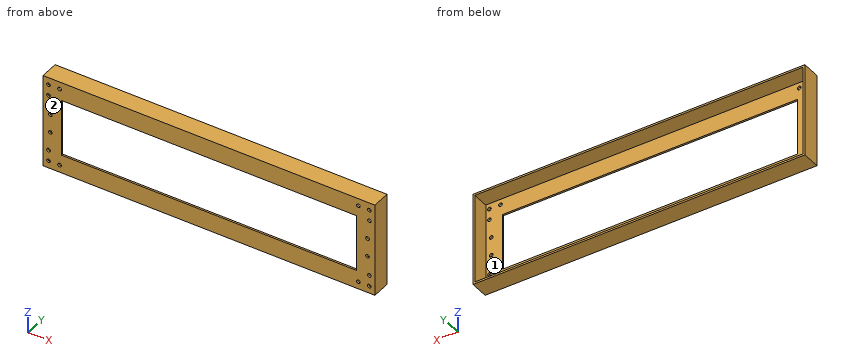
from build123d import *

# Parameters (mm, degrees)
CUT_EXTRUDE1_DEPTH      = 472.899618563
CUT_EXTRUDE1_DEPTH_BACK = 472.899618563
SKETCH5_R               = 5


with BuildPart() as part:
    # Sweep3: sweep along a path in Sketch1
    with BuildLine(Plane(origin=(0, 0, 0), x_dir=(1, 0, 0), z_dir=(0, 1, 0))) as sweep3_path:
        Line((-450, -125), (450, -125))
        Line((450, -125), (450, 125))
        Line((450, 125), (-450, 125))
        Line((-450, 125), (-450, -125))
    # Sketch2 → Sweep3 (sweep)
    with BuildSketch(Plane.XY):
        Polygon((402, -2.5), (452, -2.5), (452, 47.5), (447, 47.5), (447, 2.5), (402, 2.5), align=None)
    sweep(path=sweep3_path.line, transition=Transition.RIGHT)

    # Sketch5 → Cut-Extrude1 (cut, two sides: drawn at the far end of the back side and taken through both)
    with BuildSketch(Plane(origin=(0, 0, 0), x_dir=(1, 0, 0), z_dir=(0, 1, 0)).offset(-CUT_EXTRUDE1_DEPTH_BACK)):
        with Locations((-437, 107)):
            Circle(SKETCH5_R)
        with Locations(Location((-407, 107, 0), (0, 0, 270))):
            Circle(SKETCH5_R)
        with Locations(Location((-432, 25, 0), (0, 0, 270))):
            Circle(SKETCH5_R)
        with Locations(Location((-437, 77, 0), (0, 0, 270))):
            Circle(SKETCH5_R)
        with Locations(Location((-407, -107, 0), (0, 0, 270))):
            Circle(SKETCH5_R)
        with Locations(Location((-437, -107, 0), (0, 0, 270))):
            Circle(SKETCH5_R)
        with Locations(Location((-437, -77, 0), (0, 0, 180))):
            Circle(SKETCH5_R)
        with Locations(Location((-432, -25, 0), (0, 0, 180))):
            Circle(SKETCH5_R)
        with Locations(Location((432, -25, 0), (0, 0, 270))):
            Circle(SKETCH5_R)
        with Locations(Location((437, -77, 0), (0, 0, 270))):
            Circle(SKETCH5_R)
        with Locations(Location((437, -107, 0), (0, 0, 270))):
            Circle(SKETCH5_R)
        with Locations(Location((407, -107, 0), (0, 0, 270))):
            Circle(SKETCH5_R)
        with Locations(Location((437, 77, 0), (0, 0, 180))):
            Circle(SKETCH5_R)
        with Locations(Location((432, 25, 0), (0, 0, 180))):
            Circle(SKETCH5_R)
        with Locations(Location((407, 107, 0), (0, 0, 270))):
            Circle(SKETCH5_R)
        with Locations(Location((437, 107, 0), (0, 0, 180))):
            Circle(SKETCH5_R)
    extrude(amount=CUT_EXTRUDE1_DEPTH + CUT_EXTRUDE1_DEPTH_BACK, mode=Mode.SUBTRACT)


solid = part.part
Can you work these out from the model? Positions are in its coordinate system, mm. Face numbers are marked on the shaded views. Give positions to 0.01 mm unless a question says otherwise; leave off trailing zeros. Order: outer loops, then holes, each group sorted by start corner. A loop starts at its lowest first (then second) coordinate and runs counter-clockwise, first axis right, second up. Notation, with made-up numbers: M -1,8.25 L 55,8.25 A27 ccw 55,43.25 Z; hole C 70.25,7.25 d4. An arc over 180 degrees is marked long. One line per question, with ' | ' between items.
Item 1: We'd pull the mould along Z, two halves only. Please class the marked faces 1 and 2: released by +Z, released by -Z, zero draft, split by the parting line, or undercut.
Answer block:
face 1: undercut | face 2: zero draft
Item 2: I'm going to push flat-ended pins straight in: pin 1 Ø13 at (x, z) = (-432, 25) entering from +Y; pin 2 Ø8 at (x, z) = (-407, -107) entering from -Y; pin 3 Ø11.5 at (x, z) = (-437, -107) entering from -Y. Where does each tip first touch, or does it pass through?
Answer block:
pin 1: stops at y = 2.5 | pin 2: passes through | pin 3: stops at y = -2.5
Item 3: Suppose I cut it at A-A, the plane x = -29.5. Write out the boundary of the cut face in (y, z), then the cut area to 3 significant figures.
Answer block:
outline: M -2.5,-127 L 47.5,-127 L 47.5,-122 L 2.5,-122 L 2.5,-77 L -2.5,-77 Z; M -2.5,77 L 2.5,77 L 2.5,122 L 47.5,122 L 47.5,127 L -2.5,127 Z | area: 950 mm2
Item 4: Suppose I cut it at B-B, the plane y = 33. Write out the boundary of the cut face in (x, z).
Answer block:
outline: M -452,-127 L 452,-127 L 452,127 L -452,127 Z; hole M -447,-122 L 447,-122 L 447,122 L -447,122 Z
Item 5: Please list where these lines run through material, in increasing order: L1, parallel to X at y = 0.85, z = -25; L2, parallel to X at y = 1, z = 107; L3, parallel to X at y = 17, z = 20.
Answer block:
L1: x = -452 to -437, -427 to -402, 402 to 427, 437 to 452 | L2: x = -452 to -442, -432 to -412, -402 to 402, 412 to 432, 442 to 452 | L3: x = -452 to -447, 447 to 452
Item 6: Suppose I cut it at C-C, the plane z = 6.5. Write out the boundary of the cut face in (x, y), then the cut area to 3 significant figures.
Answer block:
outline: M -452,-2.5 L -402,-2.5 L -402,2.5 L -447,2.5 L -447,47.5 L -452,47.5 Z; M 402,-2.5 L 452,-2.5 L 452,47.5 L 447,47.5 L 447,2.5 L 402,2.5 Z | area: 950 mm2
